Can you work these out from the model? Positions are in its coordinate system, mm. Face numbers are marked on the shaded views. A direction names the side the tool comes from. Coordinates: 2 decimals unless noted, no trailing zeros. Order: outer loops, then holes, each group sorted by start corner. A loop starts at its lowest first (then second) coordinate and runs counter-clockwise, first axis right, second up. Notation, with made-up numbers: (30.25, -1) -> (64.25, -1) arc R26 ccw to (64.25, 19) -> close; hole circle Ø5 at (-27.5, 72.5). An arc over 180 degrees is marked (long way). Answer in a Markdown table with one row per item.
```python
from build123d import *

# Parameters (mm, degrees)
SKETCH1_R           = 12.665
SKETCH1_R_2         = 2.554599
SKETCH1_R_3         = 5
BOSS_EXTRUDE1_DEPTH = 14
FILLET1_R           = 4
SKETCH9_R           = 12.665
BOSS_EXTRUDE2_DEPTH = 2
SKETCH11_R          = 7.5
BOSS_EXTRUDE3_DEPTH = 2


with BuildPart() as part:
    # Sketch1 → Boss-Extrude1 (new body)
    with BuildSketch(Plane.XY):
        Polygon((20, -10), (20, 20), (-20, 20), (-20, -10), (-20, -60), (20, -60), align=None)
        Circle(SKETCH1_R, mode=Mode.SUBTRACT)
        with Locations((-15, 15)):
            Circle(SKETCH1_R_2, mode=Mode.SUBTRACT)
        with Locations((15, 15)):
            Circle(SKETCH1_R_2, mode=Mode.SUBTRACT)
        with Locations((-15, -55)):
            Circle(SKETCH1_R_2, mode=Mode.SUBTRACT)
        with Locations((15, -55)):
            Circle(SKETCH1_R_2, mode=Mode.SUBTRACT)
        with Locations((0, -34)):
            Circle(SKETCH1_R_3, mode=Mode.SUBTRACT)
    extrude(amount=BOSS_EXTRUDE1_DEPTH)

    # Fillet1
    fillet1_edges = [part.edges().sort_by_distance(p)[0] for p in [
        (-20, 20, 7),
        (20, 20, 7),
        (20, -60, 7),
        (-20, -60, 7),
    ]]
    fillet(fillet1_edges, radius=FILLET1_R)

    # Sketch9 → Boss-Extrude2 (add)
    with BuildSketch(Plane(origin=(0, 0, 0), x_dir=(-1, 0, 0), z_dir=(0, 0, -1))):
        Circle(SKETCH9_R)
    extrude(amount=-BOSS_EXTRUDE2_DEPTH)

    # Sketch11 → Boss-Extrude3 (add)
    with BuildSketch(Plane(origin=(0, 0, 0), x_dir=(-1, 0, 0), z_dir=(0, 0, -1))):
        with Locations((0, -34)):
            Circle(SKETCH11_R)
    extrude(amount=-BOSS_EXTRUDE3_DEPTH)


solid = part.part
```
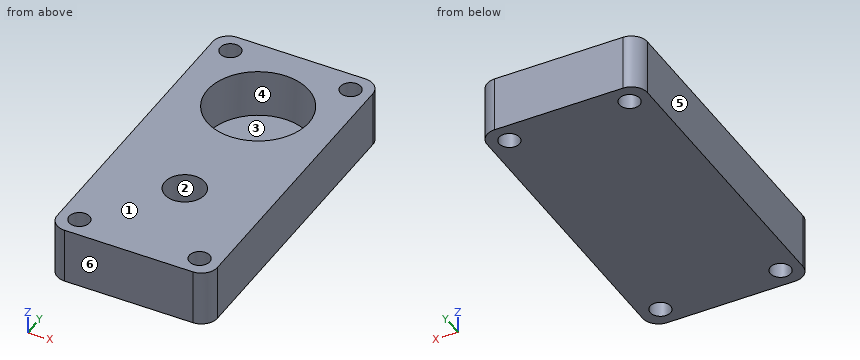
(1) Will these pins go through, and if not, where does the flat tip stop? pin 1 Ø9 at (x, y) = (0, -34) entering from +Z; pin 2 Ø3 at (x, y) = (15, -55) entering from -Z.
Response values:
| item | result |
|---|---|
| pin 1 | z = 2 |
| pin 2 | through |
(2) Suppose I cut it at B-B (x = 15). Please give me the cut outline in (y, z).
Response values:
| item | result |
|---|---|
| outline | (-60, 0) -> (-57.55, 0) -> (-57.55, 14) -> (-60, 14) -> close; (-52.45, 0) -> (12.45, 0) -> (12.45, 14) -> (-52.45, 14) -> close; (17.55, 0) -> (20, 0) -> (20, 14) -> (17.55, 14) -> close |
(3) We'd pull the mould along X, two halves only. Please class the marked faces 3, 4, 5 and 6: +X half, -X half, draft (parallel to the pull), parting line (faces both ways), or undercut.
Response values:
| item | result |
|---|---|
| face 3 | undercut |
| face 4 | undercut |
| face 5 | -X half |
| face 6 | draft |
(4) I need wall thicknesses on line 1 (Y direction, x = 15, z = 10.5); line 2 (X direction, y = -56.5, z = 5); line 3 (X direction, y = 0, z = 6) (3 decimals). Which ranges of each line are inside material? Lowest first, please. Write a range as [from, to].
Response values:
| item | result |
|---|---|
| line 1 | [-60, -57.55], [-52.45, 12.45], [17.55, 20] |
| line 2 | [-19.97, -17.07], [-12.93, 12.93], [17.07, 19.97] |
| line 3 | [-20, -12.665], [12.665, 20] |
(5) Suppose I cut it at A-A (y = 15). Please give me the cut outline in (x, z).
Response values:
| item | result |
|---|---|
| outline | (-20, 0) -> (-17.55, 0) -> (-17.55, 14) -> (-20, 14) -> close; (-12.45, 0) -> (12.45, 0) -> (12.45, 14) -> (-12.45, 14) -> close; (17.55, 0) -> (20, 0) -> (20, 14) -> (17.55, 14) -> close |
(6) Suppose I cut it at C-C (z = 11.5). Please give me the cut outline in (x, y) (3 decimals), and give its area (3 significant figures).
Response values:
| item | result |
|---|---|
| outline | (-20, -56) arc R4 ccw to (-16, -60) -> (16, -60) arc R4 ccw to (20, -56) -> (20, 16) arc R4 ccw to (16, 20) -> (-16, 20) arc R4 ccw to (-20, 16) -> close; hole circle Ø5.109 at (-15, -55); hole circle Ø5.109 at (-15, 15); hole circle Ø25.33 at (0, 0); hole circle Ø10 at (0, -34); hole circle Ø5.109 at (15, -55); hole circle Ø5.109 at (15, 15) |
| area | 2,520 mm2 |
(7) On a 3-axis mill with a long thin cutter (end or side, diameter ignored), from which of +Z, -Z, +X, -X, +Y, -Y can I reach the whole of each face in a straight line? I mean the marked faces 1 and 2. Say none if no direction works.
Response values:
| item | result |
|---|---|
| face 1 | +Z, +X, -X, +Y, -Y |
| face 2 | +Z |
(8) Suppose I cut it at D-D (z = 1). Please give me the cut outline in (x, y).
Response values:
| item | result |
|---|---|
| outline | (-20, -56) arc R4 ccw to (-16, -60) -> (16, -60) arc R4 ccw to (20, -56) -> (20, 16) arc R4 ccw to (16, 20) -> (-16, 20) arc R4 ccw to (-20, 16) -> close; hole circle Ø5.11 at (-15, -55); hole circle Ø5.11 at (-15, 15); hole circle Ø5.11 at (15, -55); hole circle Ø5.11 at (15, 15) |
